Answer from the drawing. Dimensions are ordinates in mm from the lowest x, y and z of the part. Coordinates: 2 decimals unless noted, no trailing zeros. Loops run counter-clockwise (first coordinate to the right, second up) from the corner with the lowest first, then second, coordinate; pieces in that order, holes last. Notation, with made-up numbers: (-20.75, -5) -> (7.25, -5) arc R22 ccw to (7.25, 26) -> close; hole circle Ø1 at (-24.5, 57.25). An arc over 180 degrees is marked (long way). Use a Markdown table: item, result.
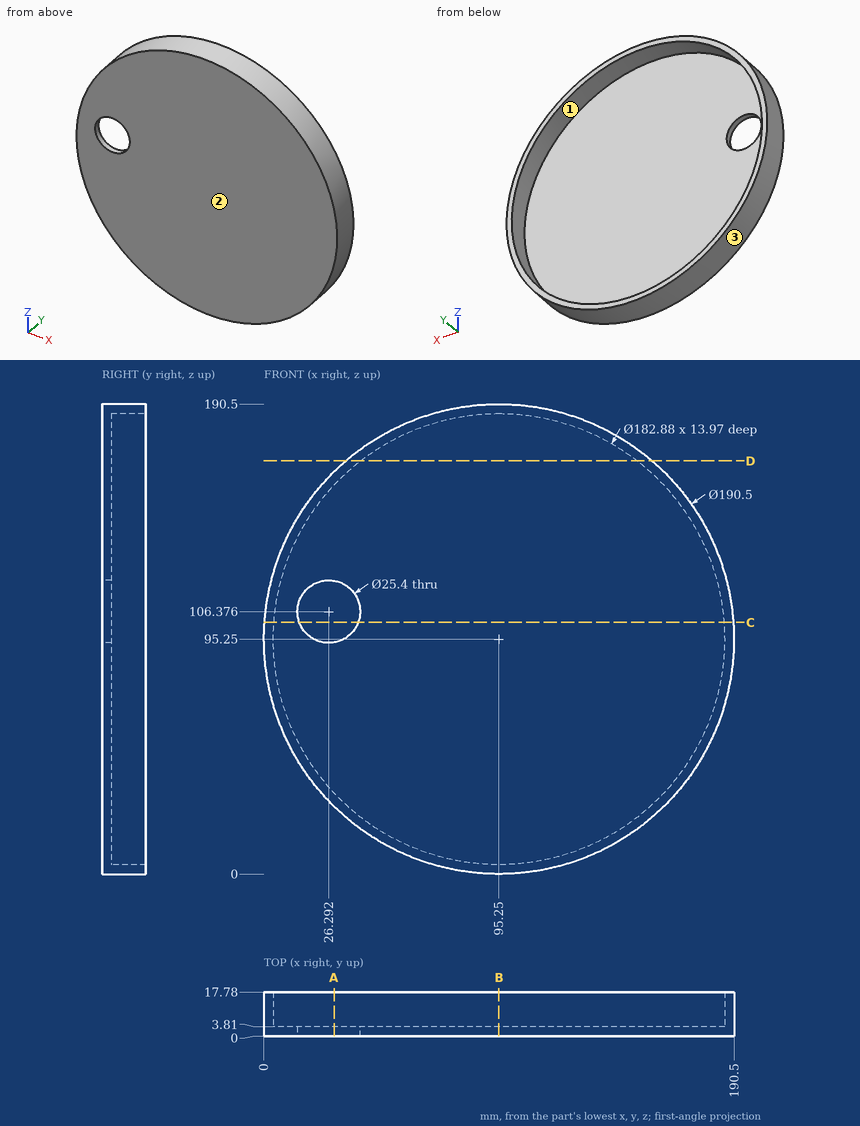
Q1. Section D-D on z = 167.5 is taken. Determine the outline of the cut face in (x, y), and give its area (3 significant figures).
Solved:
| item | result |
|---|---|
| outline | (33.18, 0) -> (157.32, 0) -> (157.32, 17.78) -> (151.3, 17.78) -> (151.3, 3.81) -> (39.2, 3.81) -> (39.2, 17.78) -> (33.18, 17.78) -> close |
| area | 641 mm² |
Q2. Determine the mould class of the marked faces 1, 2 and 3 for opening direction Z: pulls with the +Z half, pulls with the -Z half, needs draft (parallel to the pull), parting line crosses it, or undercut.
Solved:
| item | result |
|---|---|
| face 1 | undercut |
| face 2 | needs draft |
| face 3 | parting line crosses it |
Q3. Section B-B on x = 95.25 is taken. Determine the outline of the cut face in (y, z).
Solved:
| item | result |
|---|---|
| outline | (0, 0) -> (17.78, 0) -> (17.78, 3.81) -> (3.81, 3.81) -> (3.81, 186.69) -> (17.78, 186.69) -> (17.78, 190.5) -> (0, 190.5) -> close |
Q4. Given pin 1 Ø10 at (x, y) = (111, 3.5) entering from +Z; pin 2 Ø4 at (y, z) = (9.5, 120.5) entering from +X; pin 3 Ø3 at (y, z) = (8, 98.5) entering from +X, each flat-ended and moving along its own axis, determine where each tip first touches the part or whether it passes through.
Solved:
| item | result |
|---|---|
| pin 1 | z = 189.89 |
| pin 2 | x = 187.62 |
| pin 3 | x = 190.48 |
Q5. Section A-A on x = 28.5 is taken. Determine the outline of the cut face in (y, z) (1 decimal), and give its area (3 significant figures).
Solved:
| item | result |
|---|---|
| outline | (0, 27.3) -> (17.8, 27.3) -> (17.8, 32.8) -> (3.8, 32.8) -> (3.8, 93.9) -> (0, 93.9) -> close; (0, 118.9) -> (3.8, 118.9) -> (3.8, 157.7) -> (17.8, 157.7) -> (17.8, 163.2) -> (0, 163.2) -> close |
| area | 575 mm² |
Q6. Consider line 1 (Z direction, x = 93, y = 15.75); line 2 (X direction, y = 15, z = 95.25); line 3 (Y direction, x = 92.5, z = 68). Determine where each line is inside the solid, lowest interval first. Write a range as [from, to].
Solved:
| item | result |
|---|---|
| line 1 | [0.03, 3.84], [186.66, 190.47] |
| line 2 | [0, 3.81], [186.69, 190.5] |
| line 3 | [0, 3.81] |
Q7. Section C-C on z = 102 is taken. Determine the outline of the cut face in (x, y), and give its area (3 significant figures).
Solved:
| item | result |
|---|---|
| outline | (0.24, 0) -> (14.37, 0) -> (14.37, 3.81) -> (4.06, 3.81) -> (4.06, 17.78) -> (0.24, 17.78) -> close; (38.21, 0) -> (190.26, 0) -> (190.26, 17.78) -> (186.44, 17.78) -> (186.44, 3.81) -> (38.21, 3.81) -> close |
| area | 740 mm² |
